Could you check a few things on this model? Use its own coordinates, in mm. A direction names the side the tool comes from. Coordinates: 2 decimals unless noted, no trailing zeros. Loops run counter-clockwise (first coordinate to the right, second up) from the corner with the lowest first, then second, coordinate; pieces in that order, holes last. Notation, with made-up numbers: (23.25, 36.25) - (45.25, 36.25) arc R24 ccw to (45.25, 65.25) - close; hole circle Ø9 at (-8, -17.75). An arc over 180 degrees is marked (long way). One line per item, written item: value. Start each with the question number.
(1) If we section it at C-C on x = 6.5: Write out the boundary of the cut face in (y, z).
(2) On a 3-axis mill with a long thin cutter (end or side, diameter ignored), from which of +Z, -Z, +X, -X, +Y, -Y can I reach the whole of each face in a straight line? I mean faces 1 (the face through (30.976, -47, 1)), 2 (the face through (-19.343, -70.189, 1.479)). Say none if no direction works.
(3) If I drill on line 1 along X through (y, z) = (-21, 2.1); line 2 along X through (y, z) = (-73, 0.6); line 3 along Y through (x, z) = (19.5, 0.5), over which ranges is the centre line in solid material (lowest first)? Write a range as from..to.
(4) I'm going to push a flat-ended pin straight in: P1, Ø12, axis at x = -8, y = -51.5, coming from the -Z side. Where does the tip first touch, or does it pass through?
(5) If we section it at A-A on z = 1.3: Write out the boundary of the cut face in (x, y), then the cut area to 3 significant figures.
(6) If we section it at B-B on y = -63.5: Write out the boundary of the cut face in (x, z).
```python
from build123d import *

# Parameters (mm, degrees)
BOSS_EXTRUDE1_DEPTH = 3
FILLET1_START       = -1
FILLET1_DEPTH       = 5
FILLET3_R           = 8


with BuildPart() as part:
    # Sketch1 → Boss-Extrude1 (new body)
    with BuildSketch(Plane.XY):
        with BuildLine():
            Line((43.039391211, 13.180231598), (31.413296253, -9.606914519))
            ThreePointArc((31.413296253, -9.606914519), (31.087115665, -10.489967002), (30.976343732, -11.424795886))
            Line((30.976343732, -11.424795886), (30.976343732, -84.424795886))
            ThreePointArc((30.976343732, -84.424795886), (29.804770857, -87.253223011), (26.976343732, -88.424795886))
            Line((26.976343732, -88.424795886), (-4.023656268, -88.424795886))
            ThreePointArc((-4.023656268, -88.424795886), (-6.852083393, -87.253223011), (-8.023656268, -84.424795886))
            Line((-8.023656268, -84.424795886), (-8.023656268, -84.124795886))
            ThreePointArc((-8.023656268, -84.124795886), (-9.195229143, -81.296368761), (-12.023656268, -80.124795886))
            Line((-12.023656268, -80.124795886), (-19.523656268, -80.124795886))
            Line((-19.523656268, -80.124795886), (-19.523656268, -71.88053816))
            ThreePointArc((-19.523656268, -71.88053816), (-19.337683681, -70.165610877), (-18.788412372, -68.530415961))
            Line((-18.788412372, -68.530415961), (20.832065435, 17.386780739))
            ThreePointArc((20.832065435, 17.386780739), (23.784106477, 20.774647022), (28.096821539, 22.036658539))
            Line((28.096821539, 22.036658539), (43.476343732, 22.036658539))
            Line((43.476343732, 22.036658539), (43.476343732, 14.998112965))
            ThreePointArc((43.476343732, 14.998112965), (43.365571799, 14.063284081), (43.039391211, 13.180231598))
        make_face()
    extrude(amount=BOSS_EXTRUDE1_DEPTH)

    # Fillet1: read off the stored shape, not the designer's step
    # Fillet1 outline → Fillet1 (cut)
    with BuildSketch(Plane.XY.offset(FILLET1_START)):
        with BuildLine():
            ThreePointArc((-12.023656268, -80.124795886), (-11.682584861, -80.139363626), (-11.343997774, -80.182960738))
            ThreePointArc((-11.343997774, -80.182960738), (-16.768389445, -77.346578315), (-19.523656268, -71.88053816))
            Line((-19.523656268, -71.88053816), (-19.523656268, -80.124795886))
            Line((-19.523656268, -80.124795886), (-12.023656268, -80.124795886))
        make_face()
    extrude(amount=FILLET1_DEPTH, mode=Mode.SUBTRACT)

    # Fillet3
    # the kernel refuses this fillet: 8 mm, written as the material it takes off along each edge
    with BuildSketch(Plane(origin=(43.476343732, 22.036658539, -19.855037992), x_dir=(-1, 0, 0), z_dir=(0, 0, 1))) as fillet3_piece_1:
        with BuildLine():
            CenterArc((7.942015197, 8), FILLET3_R, 186.902595068, 83.097404932)
            Line((0, 7.038545575), (0, 0))
            Line((0, 0), (7.942015197, 0))
        make_face()
    extrude(amount=42.710075985, mode=Mode.SUBTRACT)


solid = part.part
```
Values:
1. outline: (-88.42, 0) - (-13.69, 0) - (-13.69, 3) - (-88.42, 3) - close
2. face 1: +Z, -Z, +X, -Y
2. face 2: +Z, -Z, -X, +Y
3. line 1: x = 3.13..30.98
3. line 2: x = -19.28..30.98
3. line 3: y = -88.42..14.5
4. P1: stops at z = 0
5. outline: (-19.52, -71.88) arc R10 ccw to (-11.34, -80.18) arc R4 cw to (-8.02, -84.12) - (-8.02, -84.42) arc R4 ccw to (-4.02, -88.42) - (26.98, -88.42) arc R4 ccw to (30.98, -84.42) - (30.98, -11.42) arc R4 cw to (31.41, -9.61) - (43.04, 13.18) arc R4 ccw to (43.48, 15) arc R8 ccw to (35.53, 22.04) - (28.1, 22.04) arc R8 ccw to (20.83, 17.39) - (-18.79, -68.53) arc R8 ccw to start
5. area: 3,740 mm2
6. outline: (-16.47, 0) - (30.98, 0) - (30.98, 3) - (-16.47, 3) - close
